from build123d import *

# Parameters (mm, degrees)
BOSS_EXTRUDE1_DEPTH      = 8.89
BOSS_EXTRUDE1_DEPTH_BACK = 8.89
SKETCH1_R                = 6.35
SKETCH2_W                = 17.78
SKETCH2_H                = 101.558108624
BOSS_EXTRUDE2_DEPTH      = 76.2


with BuildPart() as part:
    # Sketch1 → Boss-Extrude1 (new, two sides: drawn at the far end of the back side and taken through both)
    with BuildSketch(Plane.XY.offset(-BOSS_EXTRUDE1_DEPTH_BACK)):
        with BuildLine():
            Line((1.458644289, 50.779054312), (16.603324728, 50.779054312))
            Line((16.603324728, 50.779054312), (16.603324728, -50.779054312))
            Line((16.603324728, -50.779054312), (-1.458644289, -50.779054312))
            ThreePointArc((-1.458644289, -50.779054312), (-50.779054312, 1.458644289), (1.458644289, 50.779054312))
        make_face()
        Circle(SKETCH1_R, mode=Mode.SUBTRACT)
    extrude(amount=BOSS_EXTRUDE1_DEPTH + BOSS_EXTRUDE1_DEPTH_BACK)

    # Sketch2 → Boss-Extrude2 (add)
    with BuildSketch(Plane(origin=(16.603324728, 0, 0), x_dir=(0, 0, -1), z_dir=(1, 0, 0))):
        Rectangle(SKETCH2_W, SKETCH2_H)
    extrude(amount=BOSS_EXTRUDE2_DEPTH)


solid = part.part
Part model, mm, in its own coordinate system. Give positions to 0.01 mm unless a question says otherwise; leave off trailing zeros. Order: outer loops, then holes, each group sorted by start corner. A loop starts at its lowest first (then second) coordinate and runs counter-clockwise, first axis right, second up. Notation, with made-up numbers: (-34, 78.25) - (-26, 78.25) arc R31 ccw to (-26, 108.25) - close; hole circle Ø11 at (45.25, 56.25). An arc over 180 degrees is marked (long way). Use a Markdown table: item, result.
1) Saw through at D-D on x = -33. List the corners of the cut face in (y, z), plus the area to 3 significant figures.
Checked values:
| item | result |
|---|---|
| outline | (-38.62, -8.89) - (38.62, -8.89) - (38.62, 8.89) - (-38.62, 8.89) - close |
| area | 1,370 mm² |
2) Two-plate mould, pull along X, no slides. Class faces 1 (the flat face through (20, -1, -8.89)), 2 (the flat face through (92.803, 1, 0)), 3 (the cylindrical face through (-1.38, -6.2, -0.12)): +X half, -X half, draft (parallel to the pull), parting line (faces both ways), or undercut.
Checked values:
| item | result |
|---|---|
| face 1 | draft |
| face 2 | +X half |
| face 3 | undercut |
3) Saw through at B-B on x = 0. List the corners of the cut face in (y, z).
Checked values:
| item | result |
|---|---|
| outline | (-50.78, -8.89) - (-6.35, -8.89) - (-6.35, 8.89) - (-50.78, 8.89) - close; (6.35, -8.89) - (50.8, -8.89) - (50.8, 8.89) - (6.35, 8.89) - close |
4) Saw through at C-C on z = -0.75. List the corners of the cut face in (x, y), plus the area to 3 significant figures.
Checked values:
| item | result |
|---|---|
| outline | (-1.46, -50.78) - (92.8, -50.78) - (92.8, 50.78) - (1.46, 50.78) arc R50.8 ccw to start; hole circle Ø12.7 at (0, 0) |
| area | 13,400 mm² |
5) Probe L1, parallel to Y at x = 0, z = 3.75; L2, parallel to Y at x = 70.5, z = -1.5; L3, parallel to X at y = -1, z = -3.25. List the from-to ranges inside material, lowest first. Write a range as from..to.
Checked values:
| item | result |
|---|---|
| L1 | -50.78..-6.35, 6.35..50.8 |
| L2 | -50.78..50.78 |
| L3 | -50.79..-6.27, 6.27..92.8 |
6) Saw through at A-A on y = 0. List the corners of the cut face in (x, z), plus the area to 3 significant figures.
Checked values:
| item | result |
|---|---|
| outline | (-50.8, -8.89) - (-6.35, -8.89) - (-6.35, 8.89) - (-50.8, 8.89) - close; (6.35, -8.89) - (92.8, -8.89) - (92.8, 8.89) - (6.35, 8.89) - close |
| area | 2,330 mm² |
7) Flat gauge pins, fed straight in: P1, Ø10, axis at y = -34, z = -3.5, coming from the -X side; P2, Ø5, axis at x = 45, z = 7, coming from the +Y side; P3, Ø7.5, axis at x = 0, y = 0, coming from the +Z side (3 decimals); P4, Ø2, axis at y = 25.5, z = -3.5, coming from the -X side. Where does each tip first touch, or does it go through?
Checked values:
| item | result |
|---|---|
| P1 | x = -41.71 |
| P2 | y = 50.78 |
| P3 | through |
| P4 | x = -44.5 |
